Verification items for this drawing (mm, ordinates from the low corner). A direction names the side the tool comes from. Give positions to 0.01 mm unless a question says otherwise; leave off trailing zeros. Write each loop counter-clockwise with the first axis right and the second up, starting at its lowest first coordinate (ties: lowest second). Pieces come first, ordered by that corner, then holes. Notation, with made-up numbers: (64, 87.25) -> (92, 87.25) arc R26 cw to (92, 108.25) -> close; hole circle Ø1 at (-24.75, 64). An arc over 180 degrees is marked (long way). Use one line per item in the form item = value. Start each with the question number.
(1) Section check C-C, the plane y = 84. Record the cut outline in (x, z).
(2) Section check A-A, the plane x = 8. Record the cut outline in (y, z).
(3) Depth check by flat-ended pin: pin 1 Ø8 at (x, y) = (2.5, 51) entering from +Z; pin 2 Ø3 at (y, z) = (22, 5) entering from -X; pin 3 Ø4 at (y, z) = (67.45, 8) entering from -X; pin 4 Ø8 at (y, z) = (50.5, 14.5) entering from -X. Enter the tip coordinate at first touch or a pass-through.
(4) Scan lines: L1, parallel to Y at x = 3.25, z = 3.25; L2, parallel to Z at x = 7.75, y = 72.5; L3, parallel to X at y = 14, z = 7.75. Record each from-to range of solid material in increasing order.
(5) Set-up check for the marked faces 1, 2 and 3: record each of +Z, -Z, +X, -X, +Y, -Y from which the full face is reachable in a straight line by a thin tool's end or side.
(6) Section check D-D, the plane x = 4.25. Record the cut outline in (y, z), plus the area to 3 significant figures.
(7) Section check B-B, the plane z = 8. Record the cut outline in (x, y).
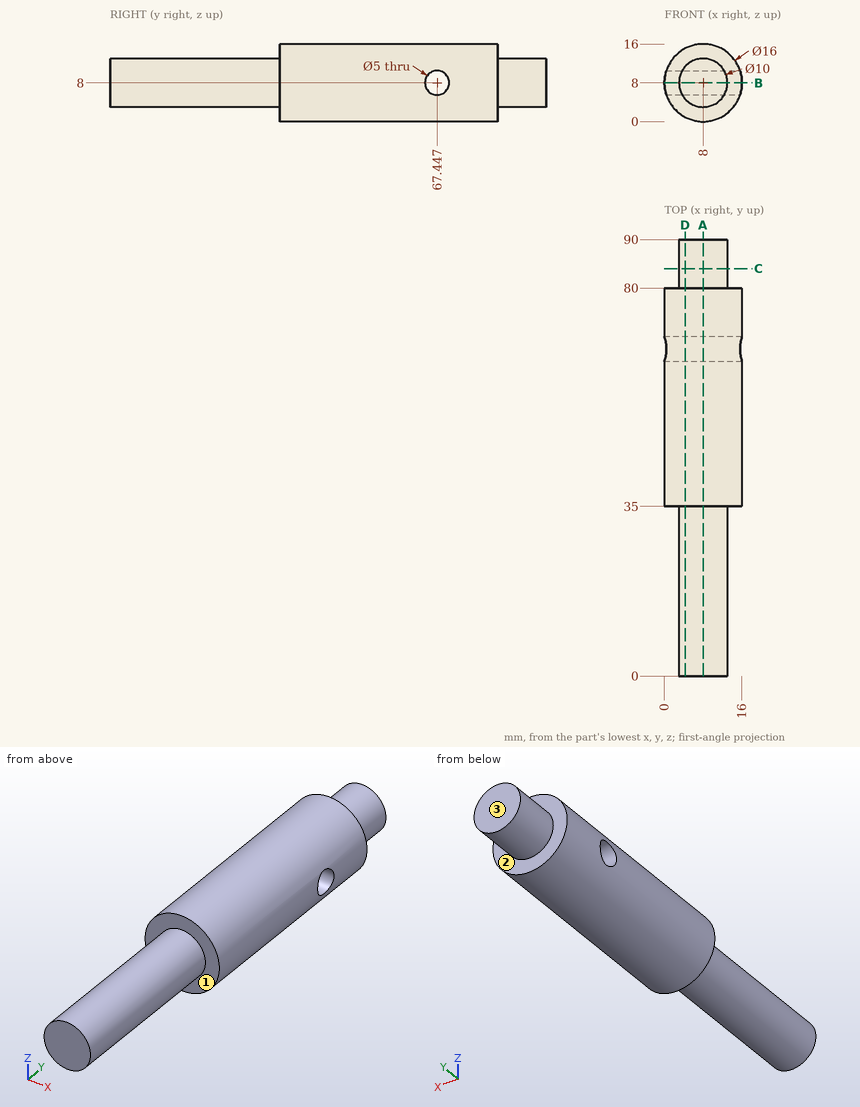
Completed:
q1.outline = circle Ø10 at (8, 8)
q2.outline = (0, 3) -> (35, 3) -> (35, 0) -> (80, 0) -> (80, 3) -> (90, 3) -> (90, 13) -> (80, 13) -> (80, 16) -> (35, 16) -> (35, 13) -> (0, 13) -> close; hole circle Ø5 at (67.45, 8)
q3.pin_1 = 15.86
q3.pin_2 = 3.23
q3.pin_3 = through
q3.pin_4 = 0.4
q4.L1 = 35 to 80
q4.L2 = 0 to 16
q4.L3 = 3.01 to 12.99
q5.face_1 = -Y
q5.face_2 = +Y
q5.face_3 = +Z, -Z, +X, -X, +Y
q6.outline = (0, 4.69) -> (35, 4.69) -> (35, 0.93) -> (80, 0.93) -> (80, 4.69) -> (90, 4.69) -> (90, 11.31) -> (80, 11.31) -> (80, 15.07) -> (35, 15.07) -> (35, 11.31) -> (0, 11.31) -> close; hole circle Ø5 at (67.45, 8)
q6.area = 914 mm²
q7.outline = (0, 35) -> (3, 35) -> (3, 0) -> (13, 0) -> (13, 35) -> (16, 35) -> (16, 64.95) -> (0, 64.95) -> close; (0, 69.95) -> (16, 69.95) -> (16, 80) -> (13, 80) -> (13, 90) -> (3, 90) -> (3, 80) -> (0, 80) -> close
